Verification items for the finished model (mm, model axes). A direction names the side the tool comes from. Coordinates: 2 decimals unless noted, no trailing zeros. Order: outer loops, then holes, each group sorted by start corner. A loop starts at its lowest first (then second) coordinate and runs counter-clockwise, first axis right, second up. Notation, with made-up numbers: M -29,7 L -1,7 A29 cw -1,30 Z; hole C -28.75,24 d1. An arc over 180 degrees is marked long. Answer as a JSON object with one key per item and string values. Group by question number.
(1) Material ranges on line 1 (Y direction, x = 0, z = 3); line 2 (Y direction, x = -2, z = -8.5); line 3 (X direction, y = 1.5, z = 5.75), recorded low to high.
(2) Cross-section at D-D (x = 3.5). Enter the section's corners in (y, z).
(3) Cross-section at C-C (z = 0.5). Enter the section's corners in (x, y), plus the area to 3 significant figures.
(4) Mould release check, pull along X, two halves, no side actions. Record for faces 3 (the face through (-1.172, 8.923, 0.175)), 4 (the face through (2, -2, 12.5)), 5 (the face through (0, -2, 6)): released by +X, released by -X, zero draft, split by the parting line, or undercut.
(5) Gauge pin test, flat ends, axial feed: pin 1 Ø8 at (y, z) = (5, 2.5) entering from +X; pin 2 Ø2.5 at (x, y) = (1.5, -0.5) entering from -Z; pin 3 Ø10 at (x, z) = (-1.5, -7.5) entering from +Y; pin 4 Ø1 at (y, z) = (-5, 0) entering from +X. Record the tip position at first contact, or that the pin passes through.
(6) Cross-section at A-A (x = 0). Enter the section's corners in (y, z).
(7) Access from +Z, -Z, +X, -X, +Y, -Y to the whole of each face (thin tool, end or side, straight path). Record for faces 1 (the face through (4, -2, -12.5)), 2 (the face through (2, -1, 0)).
from build123d import *

# Parameters (mm, degrees)
SKETCH1_R           = 9
BOSS_EXTRUDE1_DEPTH = 12.5
CUT_EXTRUDE1_START  = -12.5
SKETCH2_R           = 2
CUT_EXTRUDE1_DEPTH  = 12.5
CUT_EXTRUDE2_START  = -12.5
SKETCH3_R           = 4
CUT_EXTRUDE2_DEPTH  = 12.5


with BuildPart() as part:
    # Sketch1 → Boss-Extrude1 (new body, symmetric)
    with BuildSketch(Plane.XY):
        Circle(SKETCH1_R)
    extrude(amount=BOSS_EXTRUDE1_DEPTH, both=True)

    # Sketch2 → Cut-Extrude1 (cut)
    with BuildSketch(Plane.XY.offset(12.5).offset(CUT_EXTRUDE1_START)):
        Circle(SKETCH2_R)
    extrude(amount=CUT_EXTRUDE1_DEPTH, mode=Mode.SUBTRACT)

    # Sketch3 → Cut-Extrude2 (cut)
    with BuildSketch(Plane(origin=(0, 0, -12.5), x_dir=(-1, 0, 0), z_dir=(0, 0, -1)).offset(CUT_EXTRUDE2_START)):
        Circle(SKETCH3_R)
    extrude(amount=CUT_EXTRUDE2_DEPTH, mode=Mode.SUBTRACT)


solid = part.part
Taken from the geometry:
{
 "1": {"line 1": "y = -9 to -2, 2 to 9", "line 2": "y = -8.77 to -3.46, 3.46 to 8.77", "line 3": "x = -8.87 to -1.32, 1.32 to 8.87"},
 "2": {"outline": "M -8.29,-12.5 L -1.94,-12.5 L -1.94,0 L 1.94,0 L 1.94,-12.5 L 8.29,-12.5 L 8.29,12.5 L -8.29,12.5 Z"},
 "3": {"outline": "C 0,0 d18; hole C 0,0 d4", "area": "242 mm²"},
 "4": {"face 3": "split by the parting line", "face 4": "zero draft", "face 5": "undercut"},
 "5": {"pin 1": "stops at x = 8.94", "pin 2": "stops at z = 0", "pin 3": "stops at y = 9", "pin 4": "stops at x = 7.79"},
 "6": {"outline": "M -9,-12.5 L -4,-12.5 L -4,0 L -2,0 L -2,12.5 L -9,12.5 Z; M 2,0 L 4,0 L 4,-12.5 L 9,-12.5 L 9,12.5 L 2,12.5 Z"},
 "7": {"face 1": "-Z, +X, -X, +Y, -Y", "face 2": "-Z"}
}
